Could you check a few things on this drawing? It's one solid part, dimensions in mm from its lowest x, y, z. Give positions to 0.01 mm unless a question says otherwise; leave off trailing zeros. Write each loop counter-clockwise with the first axis right and the second up, starting at its lowest first coordinate (ties: lowest second). Pieces come first, ordered by that corner, then holes. Notation, with made-up numbers: M -32.5,38.5 L 7.5,38.5 A25 ccw 7.5,56.5 Z; hole C 46.5,55.5 d3. An arc over 180 degrees is marked long. Write each question's results on one line, items separated by ' | '. Start each with the question number.
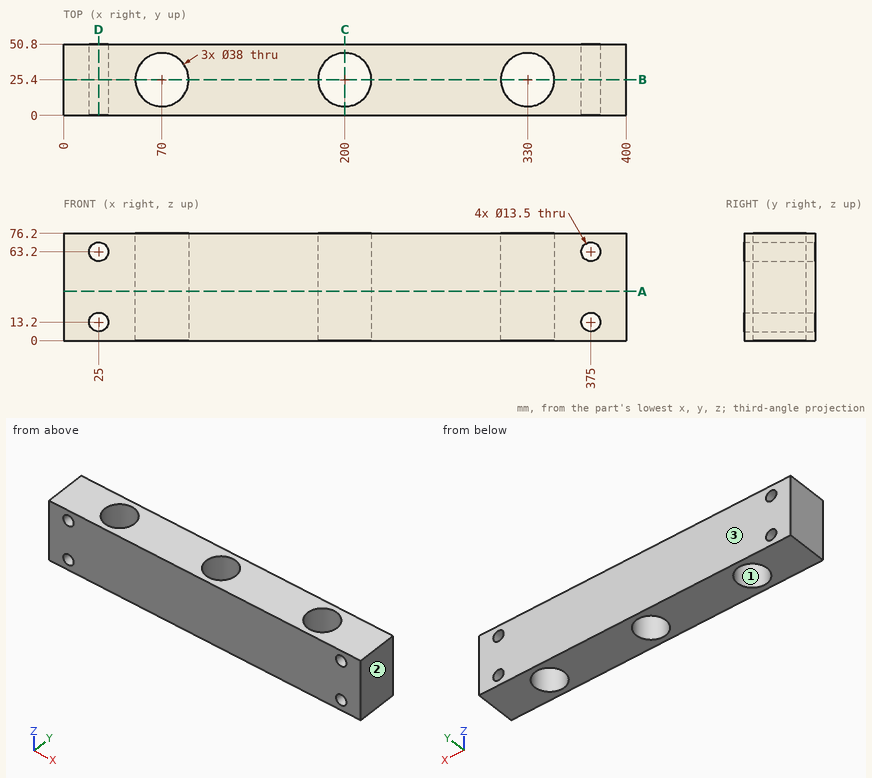
Q1. If we mould it in two halves opening along X, with no side actions, what happens to the marked faces 1, 2 and 3? For each: pulls with the +X half, pulls with the -X half, needs draft (parallel to the pull), parting line crosses it, or undercut.
Q2. If we section it at D-D (x = 25): Please give me the cut outline in (y, z).
Q3. Please list where these lines run through material, in increasing order: line 1 (X direction, y = 25, z = 30); line 2 (Z direction, x = 25, y = 32.5); line 3 (X direction, y = 19, z = 18). Write a range as [from, to].
Q4. If we section it at C-C (x = 200): Please give me the cut outline in (y, z).
Q5. If we section it at A-A (z = 35): Please give me the cut outline in (x, y), plus the area to 3 significant figures.
Q6. If we section it at B-B (y = 25.4): Please give me the cut outline in (x, z).
Determined:
1) face 1: undercut | face 2: pulls with the +X half | face 3: needs draft
2) outline: M 0,0 L 50.8,0 L 50.8,6.45 L 0,6.45 Z; M 0,19.95 L 50.8,19.95 L 50.8,56.45 L 0,56.45 Z; M 0,69.95 L 50.8,69.95 L 50.8,76.2 L 0,76.2 Z
3) line 1: x = [0, 51], [89, 181], [219, 311], [349, 400] | line 2: z = [0, 6.45], [19.95, 56.45], [69.95, 76.2] | line 3: x = [0, 20.25], [29.75, 52.11], [87.89, 182.11], [217.89, 312.11], [347.89, 370.25], [379.75, 400]
4) outline: M 0,0 L 6.4,0 L 6.4,76.2 L 0,76.2 Z; M 44.4,0 L 50.8,0 L 50.8,76.2 L 44.4,76.2 Z
5) outline: M 0,0 L 400,0 L 400,50.8 L 0,50.8 Z; hole C 70,25.4 d38; hole C 200,25.4 d38; hole C 330,25.4 d38 | area: 16,900 mm²
6) outline: M 0,0 L 51,0 L 51,76.2 L 0,76.2 Z; M 89,0 L 181,0 L 181,76.2 L 89,76.2 Z; M 219,0 L 311,0 L 311,76.2 L 219,76.2 Z; M 349,0 L 400,0 L 400,76.2 L 349,76.2 Z; hole C 25,13.2 d13.5; hole C 25,63.2 d13.5; hole C 375,13.2 d13.5; hole C 375,63.2 d13.5
